Check sheet for the modelled part. Datum: model origin and axes. Units: mm. Coordinates: 2 decimals unless noted, no trailing zeros. Loops run counter-clockwise (first coordinate to the right, second up) from the corner with the lowest first, then second, coordinate; pieces in that order, holes last. Notation, with made-up numbers: (-31, 37) -> (25, 37) arc R27 ccw to (25, 68) -> close; hole circle Ø8 at (13.5, -11). An arc over 180 degrees is marked (long way). Use one line per item in the form item = value.
from build123d import *

# Parameters (mm, degrees)
F0_R     = 13.2
F0_R_2   = 11.2
F1_DEPTH = 7


with BuildPart() as f1:
    # F0 (on Top) → F1 (new body)
    with BuildSketch(Plane.XY):
        with BuildLine():
            ThreePointArc((9.5953492139, 18.3128915938), (-1.0631566346, 14.2205026085), (-10.9263000524, 19.9711370473))
            ThreePointArc((-10.9263000524, 19.9711370473), (-11.3263382991, 7.4750183656), (-20.6571039439, -0.8466296194))
            ThreePointArc((-20.6571039439, -0.8466296194), (-13.3527241318, -5.5051193862), (-10.509713096, -13.6888092384))
            ThreePointArc((-10.509713096, -13.6888092384), (-10.8446240081, -16.6433790483), (-11.8323619992, -19.4480219384))
            ThreePointArc((-11.8323619992, -19.4480219384), (-0.8103866488, -13.5464058816), (11.06175473, -17.4662619743))
            ThreePointArc((11.06175473, -17.4662619743), (12.8468948308, -6.1895306505), (22.7586620517, -0.5231151089))
            ThreePointArc((22.7586620517, -0.5231151089), (12.1367249479, 6.071387516), (9.5953492139, 18.3128915938))
        make_face()
        Circle(F0_R, mode=Mode.SUBTRACT)
        with BuildLine():
            ThreePointArc((9.5953492139, 18.3128915938), (12.2657777907, 22.5000478532), (13.2, 27.3776184767))
            ThreePointArc((13.2, 27.3776184767), (-3.8738120313, 39.9963973537), (-10.9263000524, 19.9711370473))
            ThreePointArc((-10.9263000524, 19.9711370473), (-1.0631566346, 14.2205026085), (9.5953492139, 18.3128915938))
        make_face()
        with Locations((0, 27.3776184767)):
            Circle(F0_R_2, mode=Mode.SUBTRACT)
        with BuildLine():
            ThreePointArc((-10.509713096, -13.6888092384), (-13.3527241318, -5.5051193862), (-20.6571039439, -0.8466296194))
            ThreePointArc((-20.6571039439, -0.8466296194), (-35.6356879957, -19.3466465187), (-11.8323619992, -19.4480219384))
            ThreePointArc((-11.8323619992, -19.4480219384), (-10.8446240081, -16.6433790483), (-10.509713096, -13.6888092384))
        make_face()
        with Locations((-23.709713096, -13.6888092384)):
            Circle(F0_R_2, mode=Mode.SUBTRACT)
        with BuildLine():
            ThreePointArc((36.909713096, -13.6888092384), (32.7009901525, -4.0246001713), (22.7586620517, -0.5231151089))
            ThreePointArc((22.7586620517, -0.5231151089), (12.8468948308, -6.1895306505), (11.06175473, -17.4662619743))
            ThreePointArc((11.06175473, -17.4662619743), (25.6185019226, -26.7500697141), (36.909713096, -13.6888092384))
        make_face()
        with Locations((23.709713096, -13.6888092384)):
            Circle(F0_R_2, mode=Mode.SUBTRACT)
        Circle(F0_R)
        Circle(F0_R_2, mode=Mode.SUBTRACT)
    extrude(amount=F1_DEPTH)


solid = f1.part
(1) Section check A-A, the plane x = -25. Record the boundary of the cut face in (y, z), plus the area to 3 significant figures.
Established:
outline = (-26.83, 0) -> (-24.81, 0) -> (-24.81, 7) -> (-26.83, 7) -> close; (-2.56, 0) -> (-0.55, 0) -> (-0.55, 7) -> (-2.56, 7) -> close
area = 28.2 mm²
(2) Section check C-C, the plane z = 2. Record the boundary of the cut face in (x, y), plus the area to 3 significant figures.
Established:
outline = (-20.66, -0.85) arc R13.2 ccw (long way) to (-11.83, -19.45) arc R15.86 cw to (11.06, -17.47) arc R13.2 ccw (long way) to (22.76, -0.52) arc R15.86 cw to (9.6, 18.31) arc R13.2 ccw (long way) to (-10.93, 19.97) arc R15.86 cw to start; hole circle Ø22.4 at (-23.71, -13.69); hole circle Ø22.4 at (0, 0); hole circle Ø22.4 at (0, 27.38); hole circle Ø22.4 at (23.71, -13.69)
area = 839 mm²
(3) Scan lines: line 1 along X through (y, z) = (28, 6.25); line 2 along X through (y, z) = (-16, 1); line 3 along Y through (x, z) = (8, 0.5). Record each from-to range of solid material in increasing order.
Established:
line_1 = -13.19 to -11.18, 11.18 to 13.19
line_2 = -36.71 to -34.67, -12.75 to -8.01, 9.12 to 12.75, 34.67 to 36.71
line_3 = -15.34 to -7.84, 7.84 to 19.54, 35.22 to 37.88
(4) Mould release check, pull along X, two halves, no side actions. Record for faces 1 (the cylindrical face through (-0.99, -13.563, 3.451)), 2 (the flat face through (-8.4, -8, 7)): +X half, -X half, draft (parallel to the pull), parting line (faces both ways), or undercut.
Established:
face_1 = undercut
face_2 = draft
(5) Section check B-B, the plane y = 22.5. Record the boundary of the cut face in (x, z), plus the area to 3 significant figures.
Established:
outline = (-12.27, 0) -> (-10.08, 0) -> (-10.08, 7) -> (-12.27, 7) -> close; (10.08, 0) -> (12.27, 0) -> (12.27, 7) -> (10.08, 7) -> close
area = 30.6 mm²
(6) Section check D-D, the plane y = -15.5. Record the boundary of the cut face in (x, z).
Established:
outline = (-36.78, 0) -> (-34.76, 0) -> (-34.76, 7) -> (-36.78, 7) -> close; (-12.66, 0) -> (-7.17, 0) -> (-7.17, 7) -> (-12.66, 7) -> close; (8.29, 0) -> (12.66, 0) -> (12.66, 7) -> (8.29, 7) -> close; (34.76, 0) -> (36.78, 0) -> (36.78, 7) -> (34.76, 7) -> close
(7) Go/stop test with flat-tipped pins: P1, Ø3, axis at x = -16.5, z = 5, coming from the +Y side; P2, Ø4, axis at y = 10, z = 6, coming from the +X side; P3, Ø1, axis at y = -12, z = 6, coming from the +X side. Record where each tip stops, or that it passes through.
Established:
P1 = 2.48
P2 = 10.98
P3 = 36.86
